Design review of the part built by this model. Coordinates are the model's own, in mm. A direction names the side the tool comes from. Give positions to 0.01 mm unless a question says otherwise; leave off trailing zeros. Write each loop counter-clockwise with the first axis right and the second up, starting at its lowest first coordinate (ties: lowest second). Pieces come first, ordered by that corner, then holes. Notation, with made-up numbers: (-8, 28) -> (48, 28) arc R31 ccw to (48, 63) -> close; hole circle Ø7 at (-39, 31.5). An arc over 180 degrees is marked (long way). Use CSV: the item, a comma, the result in double quotes.
```python
from build123d import *

# Parameters (mm, degrees)
PAD_DEPTH       = 6.5
SKETCH001_R     = 16.5
PAD001_DEPTH    = 3
PAD002_DEPTH    = 34
SKETCH003_R     = 5
POCKET_DEPTH    = 30
CHAMFER_SIZE    = 1.25
SKETCH004_W     = 71
SKETCH004_H     = 50
PAD003_DEPTH    = 70
SKETCH005_R     = 32
PAD004_DEPTH    = 142
PAD005_DEPTH    = 36
PAD006_DEPTH    = 310
PAD007_DEPTH    = 6
POCKET001_DEPTH = 142.001
POCKET002_DEPTH = 422.001
SKETCH011_R     = 12
POCKET003_DEPTH = 300
SKETCH012_R     = 12
PAD008_DEPTH    = 7
CHAMFER001_SIZE = 6
FILLET_R        = 3


with BuildPart() as part:
    # Sketch → Pad (new body)
    with BuildSketch(Plane.XY):
        with BuildLine():
            Line((-22, 25), (17, 25))
            Line((17, 25), (25, 17))
            Line((25, 17), (25, -17))
            Line((17, -25), (25, -17))
            Line((17, -25), (-22, -25))
            ThreePointArc((-25, -22), (-24.12132, -24.12132), (-22, -25))
            Line((-25, -22), (-25, 22))
            ThreePointArc((-22, 25), (-24.12132, 24.12132), (-25, 22))
        make_face()
    extrude(amount=PAD_DEPTH)

    # Sketch001 (on Face10 of Pad) → Pad001 (join)
    with BuildSketch(Plane.XY.offset(6.5)):
        Circle(SKETCH001_R)
    extrude(amount=PAD001_DEPTH)

    # Sketch002 (on Face12 of Pad001) → Pad002 (join)
    with BuildSketch(Plane.XY.offset(9.5)):
        with BuildLine():
            ThreePointArc((-5.385165, 14), (-10.750761, 10.460456), (-14.142136, 5))
            Line((-14.142136, 5), (14.142136, 5))
            ThreePointArc((14.142136, 5), (10.750761, 10.460456), (5.385165, 14))
            Line((-5.385165, 14), (5.385165, 14))
        make_face()
        with BuildLine():
            Line((-14.142136, -5), (14.142136, -5))
            ThreePointArc((5.385165, -14), (10.750761, -10.460456), (14.142136, -5))
            Line((-5.385165, -14), (5.385165, -14))
            ThreePointArc((-14.142136, -5), (-10.750761, -10.460456), (-5.385165, -14))
        make_face()
    extrude(amount=PAD002_DEPTH)

    # Sketch003 (on Face14 of Pad002) → Pocket (cut)
    with BuildSketch(Plane.XZ.offset(14)):
        with Locations((0, 27.5)):
            Circle(SKETCH003_R)
        with BuildLine():
            ThreePointArc((14.387495, 34.5), (0, 43.5), (-14.387495, 34.5))
            Line((-14.387495, 34.5), (-14.387495, 44.5))
            Line((14.387495, 44.5), (-14.387495, 44.5))
            Line((14.387495, 34.5), (14.387495, 44.5))
        make_face()
    extrude(amount=-POCKET_DEPTH, mode=Mode.SUBTRACT)

    # Chamfer
    chamfer_edges = [part.edges().sort_by_distance(p)[0] for p in [
        (-16.5, 0, 9.5),
    ]]
    chamfer(chamfer_edges, length=CHAMFER_SIZE)

    # Sketch004 (on Face21 of Chamfer) → Pad003 (join)
    with BuildSketch(Plane(origin=(0, 0, 0), x_dir=(1, 0, 0), z_dir=(0, 0, -1))):
        with Locations((-10.5, 0)):
            Rectangle(SKETCH004_W, SKETCH004_H)
    extrude(amount=PAD003_DEPTH)

    # Sketch005 (on Face1 of Pad003) → Pad004 (join)
    with BuildSketch(Plane.XZ.offset(25)):
        with Locations((-22, -35)):
            Circle(SKETCH005_R)
    extrude(amount=-PAD004_DEPTH)

    # Sketch006 (on Face6 of Pad004) → Pad005 (join)
    with BuildSketch(Plane(origin=(0, 0, -70), x_dir=(1, 0, 0), z_dir=(0, 0, -1))):
        with BuildLine():
            ThreePointArc((-20.434346, -10), (22.75, 0), (-20.434346, 10))
            Line((-45.75, 10), (-20.434346, 10))
            Line((-45.75, -10), (-45.75, 10))
            Line((-20.434346, -10), (-45.75, -10))
        make_face()
    extrude(amount=PAD005_DEPTH)

    # Sketch007 (on Face27 of Pad005) → Pad006 (join)
    with BuildSketch(Plane(origin=(0, 0, -106), x_dir=(1, 0, 0), z_dir=(0, 0, -1))):
        with BuildLine():
            ThreePointArc((-16.78541, -6.5), (18, 0), (-16.78541, 6.5))
            Line((-32.5, 6.5), (-16.78541, 6.5))
            Line((-32.5, -6.5), (-32.5, 6.5))
            Line((-16.78541, -6.5), (-32.5, -6.5))
        make_face()
    extrude(amount=PAD006_DEPTH)

    # Sketch008 (on Face35 of Pad006) → Pad007 (join)
    with BuildSketch(Plane(origin=(0, 0, -416), x_dir=(1, 0, 0), z_dir=(0, 0, -1))):
        with BuildLine():
            ThreePointArc((-17.728861, -7.5), (19.25, 0), (-17.728861, 7.5))
            Line((-33.75, 7.5), (-17.728861, 7.5))
            Line((-33.75, -7.5), (-33.75, 7.5))
            Line((-17.728861, -7.5), (-33.75, -7.5))
        make_face()
    extrude(amount=PAD007_DEPTH)

    # Sketch009 (on Face1 of Pad003) → Pocket001 (cut, through all)
    with BuildSketch(Plane.XZ.offset(25)):
        with BuildLine():
            ThreePointArc((-27, -3.393039), (-46.33105, -14.21539), (-54, -35))
            Line((-54, -35), (-54, 0))
            Line((-25, 0), (-54, 0))
            Line((-25, -1.393039), (-25, 0))
            Line((-27, -3.393039), (-25, -1.393039))
        make_face()
    extrude(amount=-POCKET001_DEPTH, mode=Mode.SUBTRACT)

    # Sketch010 (on Face4 of Pad003) → Pocket002 (cut, through all)
    with BuildSketch(Plane.XY):
        Polygon((-38, -25), (-38, -18.5), (-46, -9.5), (-46, 11.5), (-55, 20.5), (-55, -25), align=None)
    extrude(amount=-POCKET002_DEPTH, mode=Mode.SUBTRACT)

    # Sketch011 (on Face5 of Pad007) → Pocket003 (cut)
    with BuildSketch(Plane(origin=(0, 0, -422), x_dir=(1, 0, 0), z_dir=(0, 0, -1))):
        Circle(SKETCH011_R)
    extrude(amount=-POCKET003_DEPTH, mode=Mode.SUBTRACT)

    # Sketch012 (on Face23 of Pad004) → Pad008 (join)
    with BuildSketch(Plane(origin=(0, 117, 0), x_dir=(-1, 0, 0), z_dir=(0, 1, 0))):
        with Locations((22, -35)):
            Circle(SKETCH012_R)
    extrude(amount=PAD008_DEPTH)

    # Chamfer001
    chamfer001_edges = [part.edges().sort_by_distance(p)[0] for p in [
        (-10, 124, -35),
    ]]
    chamfer(chamfer001_edges, length=CHAMFER001_SIZE)

    # Fillet
    fillet_edges = [part.edges().sort_by_distance(p)[0] for p in [
        (-46.33105, 117, -14.21539),
        (-1.21539, 117, -10.66895),
        (-22, 117, -67),
    ]]
    fillet(fillet_edges, radius=FILLET_R)


solid = part.part
```
(1) For line 1 along X through (y, z) = (-9, 27); line 2 along Z through (x, y) = (0, -11.25); line 3 along Z through (x, y) = (-5, -17.5), list the stretches that pass through material, from the lowest coordinate up. Write a range as [from, to].
Established:
line 1,"x = [-12, -4.97], [4.97, 12]"
line 2,"z = [-122, 22.5], [32.5, 43.5]"
line 3,"z = [-422, -416], [-106, 6.5]"
(2) Take a section at A-A (z = 27.5). Write out the cut boundary in (x, y).
Established:
outline,"(-14.14, -5) arc R15 ccw to (-5.39, -14) -> (-5, -14) -> (-5, -5) -> close; (-14.14, 5) -> (-5, 5) -> (-5, 14) -> (-5.39, 14) arc R15 ccw to start; (5, -14) -> (5.39, -14) arc R15 ccw to (14.14, -5) -> (5, -5) -> close; (5, 5) -> (14.14, 5) arc R15 ccw to (5.39, 14) -> (5, 14) -> close"
(3) Clearance check with flat-ended pins moving along their axes: pin 1 (3 mm diameter, centred on y = -22.5, z = -49, fed in from -X); pin 2 (1.5 mm diameter, centred on y = 47, z = -32, fed in from -X); pin 3 (4.5 mm diameter, centred on x = -24, z = -204, fed in from -Y). State where each tip first meets the part, or that it passes through.
Established:
pin 1,"stops at x = -38"
pin 2,"stops at x = -53.92"
pin 3,"stops at y = -6.5"
(4) Take a section at D-D (z = -35). Write out the cut boundary in (x, y), then the cut area to 3 significant figures.
Established:
outline,"(-54, 19.5) -> (-46, 11.5) -> (-46, -9.5) -> (-38, -18.5) -> (-38, -25) -> (25, -25) -> (25, 25) -> (10, 25) -> (10, 114) arc R3 ccw to (7, 117) -> (-10, 117) -> (-10, 118) -> (-16, 124) -> (-28, 124) -> (-34, 118) -> (-34, 117) -> (-51, 117) arc R3 ccw to (-54, 114) -> close"
area,"9,550 mm2"
(5) Tool access review of faces 1 (the face through (-20.44, 117.49, -23.1)), 2 (the face through (22.734, 0.855, -87.748)), 3 (the face through (23, 23, 0)), 4 (the face through (-25, 0, 2)), 5 (the face through (-25, -6.5, -259)): name each direction out of +Z, -Z, +X, -X, +Y, -Y from which nothing blocks a thin tool from reaching the whole face with its end or side.
Established:
face 1,"+Y"
face 2,"-Z"
face 3,"+Z, +X, +Y"
face 4,"+Z, -X, +Y, -Y"
face 5,"-X, -Y"
(6) Take a section at C-C (z = -256.5). Write out the cut boundary in (x, y), then the cut area to 3 significant figures.
Established:
outline,"(-32.5, -6.5) -> (-16.79, -6.5) arc R18 ccw (long way) to (-16.79, 6.5) -> (-32.5, 6.5) -> close; hole circle Ø24 at (0, 0)"
area,"759 mm2"
(7) Mouldability with a two-part tool opening along Y and no side actions: class faces 6 (the face through (13, 25, -31)), 7 (the face through (0, 5, 22)), 8 (the face through (21, -21, 3)) as +Y half, -Y half, draft (parallel to the pull), parting line (faces both ways), or undercut.
Established:
face 6,"+Y half"
face 7,"undercut"
face 8,"-Y half"
